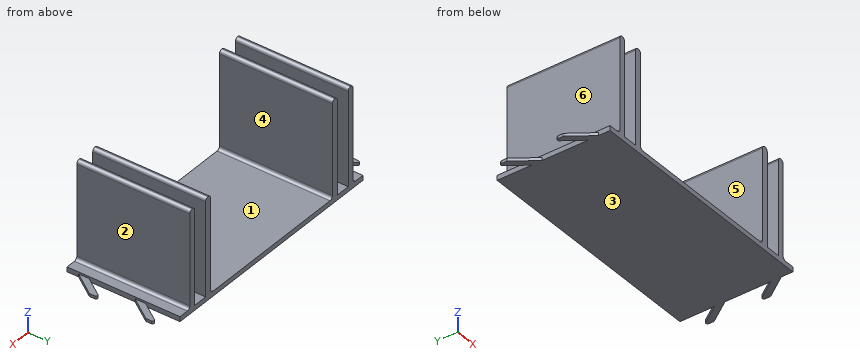
```python
from build123d import *

# Parameters (mm, degrees)
F0_W     = 4
F0_H     = 60
F1_DEPTH = 70
F2_R     = 1.99999
F3_R     = 2
F5_DEPTH = 1.8
F6_R     = 1


# Not quite as in the source:
# - a fillet or chamfer is up to 0.001 mm smaller than in the source, because OpenCascade refuses the exact size


with BuildPart() as f1:
    # F0 (on Front) → F1 (new body)
    with BuildSketch(Plane.XZ):
        Polygon((0, -20), (0, -23), (65, -23), (65, -21), (67, -21), (67, -20), (63, -20), (54, -20), (50, -20), align=None)
        Polygon((-65, -23), (0, -23), (0, -20), (-50, -20), (-54, -20), (-63, -20), (-67, -20), (-67, -21), (-65, -21), align=None)
        Polygon((65, -21), (65, -23), (71, -23), (71, -22.25), (71, -21), (67, -21), align=None)
        Polygon((-71, -23), (-65, -23), (-65, -21), (-67, -21), (-71, -21), (-71, -22.25), align=None)
        Polygon((71, -22.25), (71, -23), (75, -23), (75, -21), (71, -21), align=None)
        with Locations((52, 10)):
            Rectangle(F0_W, F0_H)
        with Locations((-52, 10)):
            Rectangle(F0_W, F0_H)
        Polygon((-75, -23), (-71, -23), (-71, -22.25), (-71, -21), (-75, -21), align=None)
        Polygon((67, -20), (67, -21), (71, -21), (75, -21), (75, -20), align=None)
        Polygon((-71, -21), (-67, -21), (-67, -20), (-75, -20), (-75, -21), align=None)
        with Locations((65, 10)):
            Rectangle(F0_W, F0_H)
        with Locations((-65, 10)):
            Rectangle(F0_W, F0_H)
    extrude(amount=F1_DEPTH)

    # F2 (radius 2 in the source; OpenCascade refuses exactly that, so slightly less here)
    f2_edges = [f1.edges().sort_by_distance(p)[0] for p in [
        (-67, -35, 40),
        (-63, -35, 40),
        (-54, -35, 40),
        (-50, -35, 40),
        (54, -35, 40),
        (50, -35, 40),
        (63, -35, 40),
        (67, -35, 40),
    ]]
    fillet(f2_edges, radius=F2_R)

    # F3
    f3_edges = [f1.edges().sort_by_distance(p)[0] for p in [
        (-50, -35, -20),
        (50, -35, -20),
        (-67, -35, -20),
        (67, -35, -20),
    ]]
    fillet(f3_edges, radius=F3_R)

    # F4 (on face) → F5 (join)
    with BuildSketch(Plane(origin=(0, 0, -23), x_dir=(1, 0, 0), z_dir=(0, 0, -1))):
        Polygon((-85, 42.1), (-75, 56.3814800674), (-75, 62.9), (-85, 48.6185199326), align=None)
        Polygon((-75, 21.3814800674), (-75, 27.9), (-85, 13.6185199326), (-85, 7.1), align=None)
        Polygon((85, 13.6185199326), (75, 27.9), (75, 21.3814800674), (85, 7.1), align=None)
        Polygon((75, 62.9), (75, 56.3814800674), (85, 42.1), (85, 48.6185199326), align=None)
    extrude(amount=-F5_DEPTH)

    # F6
    f6_edges = [f1.edges().sort_by_distance(p)[0] for p in [
        (85, -42.1, -22.1),
        (85, -7.1, -22.1),
        (85, -13.61852, -22.1),
        (85, -48.61852, -22.1),
        (-85, -7.1, -22.1),
        (-85, -13.61852, -22.1),
        (-85, -42.1, -22.1),
        (-85, -48.61852, -22.1),
    ]]
    fillet(f6_edges, radius=F6_R)


solid = f1.part
```
Input: part model. Units: mm. Frame: model coordinates. Face numbers are marked on the shaded views. A direction names the side the tool comes from. Coordinates: 2 decimals unless noted, no trailing zeros. Write each loop counter-clockwise with the first axis right and the second up, starting at its lowest first coordinate (ties: lowest second). Pieces come first, ordered by that corner, then holes. Notation, with made-up numbers: (42, 13) - (84, 13) arc R11 ccw to (84, 27) - close; hole circle Ø9 at (56, 86.25). An arc over 180 degrees is marked (long way). Put each result on its own line as item: value. Start each with the question number.
1) Cut plane A-A (z = 28). Return the cut outline in (x, y).
2) Cut plane C-C (x = 41). Return the cut outline in (y, z).
3) Mould query, pull axis X, two halves, no side actions, for the marked faces 3, 4, 5 and 6. Classes: pulls with the +X half, pulls with the -X half, needs draft (parallel to the pull), parting line crosses it, or undercut.
4) Contact query for flat-ended pins moving along their axis: pin 1 (3 mm diameter, centred on x = 81, y = -16.5, fed in from +Z); pin 2 (5 mm diameter, centred on x = -71.5, y = -49, fed in from +Z); pin 3 (4 mm diameter, centred on x = -47, y = -45, fed in from +Z). Output: stop coordinate, or through.
5) Reachability of the marked faces 1 and 2 from +Z, -Z, +X, -X, +Y, -Y: full face, straight path, thin tool, end or side. Return the list, or none.
6) Ray query, L1, parallel to X at y = -19.5, z = 37; L2, parallel to Z at x = -43, y = -45; L3, parallel to Z at x = -68.5, y = -48. Return the intervals inside material, ascending.
Resolved:
1. outline: (-67, -70) - (-63, -70) - (-63, 0) - (-67, 0) - close; (-54, -70) - (-50, -70) - (-50, 0) - (-54, 0) - close; (50, -70) - (54, -70) - (54, 0) - (50, 0) - close; (63, -70) - (67, -70) - (67, 0) - (63, 0) - close
2. outline: (-70, -23) - (0, -23) - (0, -20) - (-70, -20) - close
3. face 3: needs draft
3. face 4: undercut
3. face 5: undercut
3. face 6: pulls with the -X half
4. pin 1: stops at z = -21.2
4. pin 2: stops at z = -20
4. pin 3: stops at z = -19.73
5. face 1: +Z, +Y, -Y
5. face 2: +Z, +X, +Y, -Y
6. L1: x = -67 to -63, -54 to -50, 50 to 54, 63 to 67
6. L2: z = -23 to -20
6. L3: z = -23 to -19.94
